Here's how the part is built. I have some questions about the finished solid (model axes, mm). A direction names the side the tool comes from. Coordinates: 2 decimals unless noted, no trailing zeros. Write each loop counter-clockwise with the first axis right and the second up, starting at its lowest first coordinate (ties: lowest second). Pieces come first, ordered by that corner, then holes.
(1) Thinking about a two-plate mould opening in Z: for faces 1 (the flat face through (-1.09, -0.51, -0.86)), 2 (the flat face through (8, 0, 0)), 3 (the cylindrical face through (3.84, -1.5, -0.07)), which applies, released by +Z, released by -Z, zero draft, split by the parting line, or undercut?
(2) Imagine slicing it at B-B, the plane x = 1.5. List the corners of the cut face in (y, z) for me.
(3) Please list where these lines run through material, in increasing order: probe 1 along Y at (x, z) = (-0.5, 0.65); probe 2 along Y at (x, z) = (0.25, -0.05).
(4) Imagine slicing it at A-A, the plane x = -0.25. List the corners of the cut face in (y, z) for me, plus the area to 3 significant figures.
(5) For pin 1 Ø0.6 at (x, z) = (-1, 0) entering from +Y; pin 2 Ø2 at (y, z) = (-0.5, -1.5) entering from +X; pin 3 Ø1.5 at (x, z) = (2, -1) entering from +Y; pin 4 Ø1.5 at (y, z) = (-2, 2) entering from +X, each with a flat end and sliding along its axis, tell me the tip position at first contact or that it passes through.
(6) Which directions (+Z, -Z, +X, -X, +Y, -Y) give clear straight access to the entire face, cutting with the end or side of a thin tool? Please do faces 4 (the cylindrical face through (-0.193, -2.262, 1.734)), 5 (the flat face through (-1, 1, 0)), 6 (the flat face through (0, 0, -2)).
Autodesk Inventor part; units mm, degrees
ref_plane "Work Plane1" through (30, 0, 0) normal (0, -0.5, 0.866) x (1, 0, 0)
ref_plane "YZ Plane" through (0, 0, 0) normal (1, 0, 0) x (0, 1, 0)
ref_plane "XZ Plane" through (0, 0, 0) normal (0, 1, 0) x (-1, 0, 0)
sketch "Sketch1" plane through (0, 0, 0) normal (0, 0, 1) x (1, 0, 0)
  line L0 (0.0567, 0) -> (8, 0)
  line L1 (8, 0) -> (8, 1.5)
  line L2 (8, 1.5) -> (1, 1.5)
  line L3 (1, 1.5) -> (0.6933, 1.5)
  line L4 (0.6933, 1.5) -> (0, 1.5)
  line L5 (0, 1.5) -> (0, 2.85)
  line L6 (0, 2.85) -> (-1.65, 2.85)
  line L7 (-1.65, 2.85) -> (-1.65, 1.1547)
  line L8 (-1.65, 1.1547) -> (-0.61, 1.1547)
  line L9 (-0.61, 1.1547) -> (0.0567, 0)
  line L10 (-3.58, 0) -> (9.93, 0)
  line L11 (0, -0.57) -> (0, 3.42)
  line L12 (1, 1.5) -> (0, 1.5) construction
  dimension "d0" = 7
  dimension "d1" = 0.3067
  dimension "d2" = 1.65
  dimension "d3" = 1.04
  dimension "d4" = 60
  dimension "d5" = 3
  dimension "d6" = 3
  dimension "d7" = 2.3094
  dimension "d8" = 5.7
  dimension "d19" = 8
revolve "Body" add sketch "Sketch1" angle 360 about axis through (0.0567, 0, 0) along (1, 0, 0) contours L9 L11 L4 L3 L2 L1 L0 | L9 L8 L7 L6 L5 L11
sketch "Sketch2" plane through (-1.65, 0, 0) normal (-1, 0, 0) x (0, 0, 1)
  circle A0 centre (0, 0) radius 1.1547
  line L0 (0, -3.99) -> (0, 3.99)
  line L1 (-3.99, 0) -> (3.99, 0)
  line L2 (1.1547, 0) -> (0.5774, -1)
  line L3 (0.5774, -1) -> (-0.5774, -1)
  line L4 (-0.5774, -1) -> (-1.1547, 0)
  line L5 (-1.1547, 0) -> (-0.5774, 1)
  line L6 (-0.5774, 1) -> (0.5774, 1)
  line L7 (0.5774, 1) -> (1.1547, 0)
extrude "Slot" add sketch "Sketch2" against normal up to next contours L7 A0 | A0 L2 | L6 L0 A0 | A0 L0 L3 | L0 L6 A0 | A0 L3 L0 | L4 A0 | A0 L5
fillet "Fillet1" radius 1.27 1 edges at (-1.65, -2.85, 0)
thread "Thread"
chamfer "Chamfer1" distance 0.3067 distance2 0.3067 1 edges at (8, -1.5, 0) measured on face at (8, 0.5539, 0.4443)
fillet "Fillet2" radius 0.1 1 edges at (0, -1.5, 0)
ref_plane "Work Plane1" through (30, 0, 0) normal (0, -0.5, 0.866) x (1, 0, 0)
equation "\"d0\" = GEL"
equation "\"d1\" = GAL"
equation "\"d2\" = KOH"
equation "\"d3\" = INTI"
equation "\"d5\" = GD"
equation "\"d6\" = BDM"
equation "\"d7\" = 1.1547 * SW"
equation "\"d8\" = KOD"
equation "\"d19\" = NLG"
equation "\"d16\" = RR"
equation "\"d12\" = GEL"
equation "\"d14\" = -0.5 * SPD + 0.5 * GD"
equation "\"d15\" = GUL"
equation "\"d29\" = R"
equation "\"GD\" = NND"
equation "\"NLG\" = 8"
equation "\"GEL\" = 7"
equation "\"KOD\" = 5.7"
equation "\"KOH\" = 1.65"
equation "\"INTI\" = 1.04"
equation "\"GAL\" = 0.61345 * PTC"
equation "\"GUL\" = 0.61345 * PTC"
equation "\"BDM\" = NND"
equation "\"SW\" = 2"
equation "\"RR\" = 1.27"
equation "\"SPD\" = 2.38655"
equation "\"d28\" = R"
equation "\"R\" = 0.1"
equation "\"TOA\" = 30deg"
equation "\"THREADDIA\" = 3"
equation "\"KOD1\" = KOD - 2 * RR"
equation "\"PTC\" = 0.5"
equation "\"NND\" = 3"
equation "\"E0\" = 1.155 * SW"
equation "\"GD1\" = THREADDIA - 1.2269 * PTC"
properties part number "ANSI B18.3.4M - M3 x 0.5 x 8, FHSBHCSM" material "Steel, Mild"
Recorded:
1. face 1: undercut
1. face 2: zero draft
1. face 3: split by the parting line
2. outline: circle Ø3 at (0, 0)
3. probe 1: y = -2.77 to -0.71, 0.71 to 2.77
3. probe 2: y = -1.5 to 1.5
4. outline: circle Ø5.7 at (0, 0); hole circle Ø1.06 at (0, 0)
4. area: 24.6 mm2
5. pin 1: stops at y = 2.81
5. pin 2: stops at x = 8
5. pin 3: stops at y = 1.48
5. pin 4: stops at x = 0
6. face 4: +X, -X
6. face 5: -X
6. face 6: +X
